```python
from build123d import *
from build123d import SkipClean  # not in build123d's __all__

# Parameters (mm, degrees)
F0_W      = 55
F0_H      = 31
F2_DEPTH  = 10
F1_W      = 51
F1_H      = 27
F3_DEPTH  = 11
F4_DEPTH  = 8
F5_W      = 51
F5_H      = 2
F6_DEPTH  = 6
F7_W      = 2
F7_H      = 23
F8_DEPTH  = 6
F10_DEPTH = 6
F11_DEPTH = 6


with BuildPart() as f2:
    # F0 (on Top) → F2 (new body)
    with BuildSketch(Plane.XY):
        with Locations((2.9806493223, 1.209073022)):
            Rectangle(F0_W, F0_H)
    extrude(amount=F2_DEPTH)

    # F1 (on face) → F3 (join)
    with BuildSketch(Plane.XY):
        Polygon((-22.5115198195, 15.6954657286), (-23.5115198195, 15.6954657286), (-23.5115198195, -13.3045342714), (29.4884801805, -13.3045342714), (29.4884801805, 15.6954657286), align=None)
        with Locations((2.9884801805, 1.1954657286)):
            Rectangle(F1_W, F1_H, mode=Mode.SUBTRACT)
    extrude(amount=F3_DEPTH)

    # F4 (cut): a face of the model
    f4_faces = [f2.faces().sort_by_distance(p)[0] for p in [
        (2.9884801805, 1.1954657286, 10),
    ]]
    extrude(f4_faces, amount=-F4_DEPTH, mode=Mode.SUBTRACT)

    # F5 (on face) → F6 (join)
    with BuildSketch(Plane.XY.offset(2)):
        with Locations((2.9884801805, 13.6954657286)):
            Rectangle(F5_W, F5_H)
        with Locations((2.9884801805, -11.3045342714)):
            Rectangle(F5_W, F5_H)
    extrude(amount=F6_DEPTH)

    # F7 (on face) → F8 (join)
    with BuildSketch(Plane.XY.offset(2)):
        with Locations((27.4884801805, 1.1954657286)):
            Rectangle(F7_W, F7_H)
        with Locations((-21.5115198195, 1.1954657286)):
            Rectangle(F7_W, F7_H)
    extrude(amount=F8_DEPTH)

    # F9 (on face) → F10 (join)
    with BuildSketch(Plane.XY.offset(8)):
        with BuildLine():
            ThreePointArc((-20.5115198195, 9.6954657286), (-18.3901994759, 10.5741453851), (-17.5115198195, 12.6954657286))
            Line((-17.5115198195, 12.6954657286), (-18.5115198195, 12.6954657286))
            ThreePointArc((-18.5115198195, 12.6954657286), (-19.0973062571, 11.2812521663), (-20.5115198195, 10.6954657286))
            Line((-20.5115198195, 10.6954657286), (-20.5115198195, 9.6954657286))
        make_face()
        with BuildLine():
            ThreePointArc((-17.5115198195, -10.3045342714), (-18.3901994759, -8.1832139278), (-20.5115198195, -7.3045342714))
            Line((-20.5115198195, -7.3045342714), (-20.5115198195, -8.3045342714))
            ThreePointArc((-20.5115198195, -8.3045342714), (-19.0973062571, -8.890320709), (-18.5115198195, -10.3045342714))
            Line((-18.5115198195, -10.3045342714), (-17.5115198195, -10.3045342714))
        make_face()
        with BuildLine():
            Line((26.4884801805, -8.3045342714), (26.4884801805, -7.3045342714))
            ThreePointArc((26.4884801805, -7.3045342714), (24.3671598369, -8.1832139278), (23.4884801805, -10.3045342714))
            Line((23.4884801805, -10.3045342714), (24.4884801805, -10.3045342714))
            ThreePointArc((24.4884801805, -10.3045342714), (25.0742666181, -8.890320709), (26.4884801805, -8.3045342714))
        make_face()
        with BuildLine():
            Line((24.4884801805, 12.6954657286), (23.4884801805, 12.6954657286))
            ThreePointArc((23.4884801805, 12.6954657286), (24.3671598369, 10.5741453851), (26.4884801805, 9.6954657286))
            Line((26.4884801805, 9.6954657286), (26.4884801805, 10.6954657286))
            ThreePointArc((26.4884801805, 10.6954657286), (25.0742666181, 11.2812521663), (24.4884801805, 12.6954657286))
        make_face()
    extrude(amount=-F10_DEPTH)

    # F9 (on face) → F11 (cut)
    with BuildSketch(Plane.XY.offset(8)):
        with BuildLine():
            Line((-20.5115198195, 12.6954657286), (-18.5115198195, 12.6954657286))
            ThreePointArc((-18.5115198195, 12.6954657286), (-19.0973062461, 14.10967928), (-20.5115197883, 14.6954657286))
            ThreePointArc((-20.5115197883, 14.6954657286), (-21.9257333708, 14.1096793021), (-22.5115198195, 12.6954657286))
            ThreePointArc((-22.5115198195, 12.6954657286), (-21.9257333819, 11.2812521663), (-20.5115198195, 10.6954657286))
            Line((-20.5115198195, 10.6954657286), (-20.5115198195, 12.6954657286))
        make_face()
        with BuildLine():
            Line((-20.5115198195, -10.3045342714), (-20.5115198195, -8.3045342714))
            ThreePointArc((-20.5115198195, -8.3045342714), (-21.9257333819, -8.890320709), (-22.5115198195, -10.3045342714))
            ThreePointArc((-22.5115198195, -10.3045342714), (-21.9257333819, -11.7187478337), (-20.5115198195, -12.3045342714))
            ThreePointArc((-20.5115198195, -12.3045342714), (-19.0973062571, -11.7187478337), (-18.5115198195, -10.3045342714))
            Line((-18.5115198195, -10.3045342714), (-20.5115198195, -10.3045342714))
        make_face()
        with BuildLine():
            ThreePointArc((28.4884801805, -10.3045342714), (27.9026937429, -8.890320709), (26.4884801805, -8.3045342714))
            Line((26.4884801805, -8.3045342714), (26.4884801805, -10.3045342714))
            Line((26.4884801805, -10.3045342714), (24.4884801805, -10.3045342714))
            ThreePointArc((24.4884801805, -10.3045342714), (25.0742666181, -11.7187478337), (26.4884801805, -12.3045342714))
            ThreePointArc((26.4884801805, -12.3045342714), (27.9026937429, -11.7187478337), (28.4884801805, -10.3045342714))
        make_face()
        with BuildLine():
            ThreePointArc((26.4884801805, 14.6954657286), (25.0742666181, 14.109679291), (24.4884801805, 12.6954657286))
            Line((24.4884801805, 12.6954657286), (26.4884801805, 12.6954657286))
            Line((26.4884801805, 12.6954657286), (26.4884801805, 10.6954657286))
            ThreePointArc((26.4884801805, 10.6954657286), (27.9026937429, 11.2812521663), (28.4884801805, 12.6954657286))
            ThreePointArc((28.4884801805, 12.6954657286), (27.9026937429, 14.109679291), (26.4884801805, 14.6954657286))
        make_face()
    with SkipClean():  # cleaning this boolean's faces spoils the solid; the shape is the same uncleaned
        extrude(amount=-F11_DEPTH, mode=Mode.SUBTRACT)


solid = f2.part
```
Read the model definition and answer for the solid it produces. Units are mm, in the model's axes. A direction names the side the tool comes from. Round coordinates to 2 decimals unless told otherwise and drop trailing zeros. Write each loop counter-clockwise with the first axis right and the second up, starting at its lowest first coordinate (ties: lowest second). Pieces come first, ordered by that corner, then holes. Notation, with made-up numbers: (-8.75, 1) - (41.25, 1) arc R13 cw to (41.25, 8) - close; hole circle Ø9 at (85.25, -14). An arc over 180 degrees is marked (long way). One line per item, written item: value.
Q1. Straight lines are drawn through the part: line 1 (X direction, y = 12.5, z = 3.75); line 2 (Y direction, x = -14, z = 7.75); line 3 (Y direction, x = -13.5, z = 8.5). For each, find the intervals that lie inside material, in ascending order. Write a range as from..to.
The answers:
line 1: x = -24.52..-22.5, -18.52..-17.52, 23.49..24.5, 28.48..30.48
line 2: y = -14.29..-10.3, 12.7..16.71
line 3: y = -14.29..-12.3, 14.7..16.71
Q2. Find section B-B (z = 8.75). Determine the outline of the cut face in (x, y).
The answers:
outline: (-24.52, -14.29) - (30.48, -14.29) - (30.48, 16.71) - (-24.52, 16.71) - close; hole (-22.51, -12.3) - (28.49, -12.3) - (28.49, 14.7) - (-22.51, 14.7) - close
Q3. For a pull along Y with two mould halves and no side action, classify faces 1 (the cylindrical face through (24.39, -8.16, 5.04)), 2 (the flat face through (3.4, 15.695, 10.5)), 3 (the flat face through (3, 12.695, 5)), 4 (the flat face through (-24.519, 1, 5)) as pulls with the +Y half, pulls with the -Y half, needs draft (parallel to the pull), parting line crosses it, or undercut.
The answers:
face 1: undercut
face 2: pulls with the +Y half
face 3: undercut
face 4: needs draft
Q4. Which of the six approach directions +Z, -Z, +X, -X, +Y, -Y give full straight-line access (tool end or side, diameter ignored) to faces 5 (the flat face through (26, -10, 2)), 6 (the flat face through (2.6, -13.305, 10.5)), 7 (the flat face through (-23.512, 1.4, 10.5))?
The answers:
face 5: +Z
face 6: +Z, +X, -X, -Y
face 7: +Z, -X, +Y, -Y
Q5. Find section D-D (x = 18.5). Determine the outline of the cut face in (y, z).
The answers:
outline: (-14.29, 0) - (16.71, 0) - (16.71, 10) - (15.7, 10) - (15.7, 11) - (14.7, 11) - (14.7, 8) - (12.7, 8) - (12.7, 2) - (-10.3, 2) - (-10.3, 8) - (-12.3, 8) - (-12.3, 11) - (-13.3, 11) - (-13.3, 10) - (-14.29, 10) - close
Q6. Find section C-C (y = 9). Determine the outline of the cut face in (x, z).
The answers:
outline: (-24.52, 0) - (30.48, 0) - (30.48, 10) - (29.49, 10) - (29.49, 11) - (28.49, 11) - (28.49, 8) - (26.49, 8) - (26.49, 2) - (-20.51, 2) - (-20.51, 8) - (-22.51, 8) - (-22.51, 11) - (-23.51, 11) - (-23.51, 10) - (-24.52, 10) - close
Q7. Find section A-A (z = 5). Determine the outline of the cut face in (x, y), and give its area (3 significant figures).
The answers:
outline: (-24.52, -14.29) - (30.48, -14.29) - (30.48, 16.71) - (-24.52, 16.71) - close; hole circle Ø4 at (-20.51, -10.3); hole circle Ø4 at (-20.51, 12.7); hole (-20.51, -7.3) arc R3 cw to (-17.51, -10.3) - (23.49, -10.3) arc R3 cw to (26.49, -7.3) - (26.49, 9.7) arc R3 cw to (23.49, 12.7) - (-17.51, 12.7) arc R3 cw to (-20.51, 9.7) - close; hole circle Ø4 at (26.49, -10.3); hole circle Ø4 at (26.49, 12.7)
area: 602 mm2
Q8. Each of these flat-tipped pins is pushed along its axis until it touches: P1, Ø11.5, axis at x = 1, y = 6, coming from the +Z side; P2, Ø1, axis at x = -21.5, y = 14, coming from the +Z side. Where does it stop, or does it pass through?
The answers:
P1: stops at z = 2
P2: stops at z = 8
